from build123d import *
from OCP.BRepFilletAPI import BRepFilletAPI_MakeChamfer

# Parameters (mm, degrees)
BOSS_EXTRUDE1_DEPTH      = 25
BOSS_EXTRUDE1_DEPTH_BACK = 25
CUT_EXTRUDE1_DEPTH       = 25
BOSS_EXTRUDE3_DEPTH      = 20
CHAMFER2_SIZE            = 10
CHAMFER2_SIZE_2          = 0.5
SKETCH5_R                = 4
CUT_EXTRUDE4_DEPTH       = 20
SKETCH6_R                = 2.25
CUT_EXTRUDE5_DEPTH       = 20
CUT_EXTRUDE6_DEPTH       = 30
CUT_EXTRUDE6_DEPTH_BACK  = 20
SKETCH7_R                = 2.25
SKETCH8_R                = 4
CUT_EXTRUDE7_DEPTH       = 20
CUT_EXTRUDE10_DEPTH      = 10
CUT_EXTRUDE10_DEPTH_BACK = 10
SKETCH10_R               = 1.875
SKETCH10_9_R             = 3
SKETCH10_9_R_2           = 1.875
CUT_EXTRUDE11_DEPTH      = 20
CHAMFER3_START           = -141.531055451
CHAMFER3_DEPTH           = 67.531055451
CHAMFER4_SIZE            = 5
CHAMFER5_START           = 49.569652266
CHAMFER5_DEPTH           = 20.503333196
CHAMFER5_START_2         = -70.072985462
CHAMFER5_2_DEPTH         = 20.503333196


with BuildPart() as part:
    # Sketch1 → Boss-Extrude1 (new, two sides: drawn at the far end of the back side and taken through both)
    with BuildSketch(Plane(origin=(0, 0, 0), x_dir=(0, 0, -1), z_dir=(1, 0, 0)).offset(-BOSS_EXTRUDE1_DEPTH_BACK)):
        Polygon((-106.218311965, -85.648642757), (-56.372445278, -89.571597544), (-57.980856741, -110.008402885), (-53, -105), (-53, -65), (-73, -65), (-105.747557391, -79.667138755), align=None)
    extrude(amount=BOSS_EXTRUDE1_DEPTH + BOSS_EXTRUDE1_DEPTH_BACK)

    # Sketch2 → Cut-Extrude1 (cut)
    with BuildSketch(Plane(origin=(0, -65, 0), x_dir=(1, 0, 0), z_dir=(0, 1, 0))):
        Polygon((16.25, -106.218311965), (16.25, -73), (25, -63), (25, -106.218311965), align=None)
        Polygon((-25, -106.218311965), (-16.25, -106.218311965), (-16.25, -73), (-25, -63), align=None)
    extrude(amount=-CUT_EXTRUDE1_DEPTH, mode=Mode.SUBTRACT)

    # Sketch3 → Boss-Extrude3 (add)
    with BuildSketch(Plane(origin=(0, -93.429506703, 7.353061645), x_dir=(1, 0, 0), z_dir=(0, -0.9969173337331282, 0.07845909572784136))):
        Polygon((10.25, 99.170961297), (10.25, 49.170961297), (25, 49.170961297), (25, 55.819009733), (16.25, 65.849931718), (16.25, 99.170961297), align=None)
        Polygon((-10.25, 99.170961297), (-10.25, 49.170961297), (-25, 49.170961297), (-25, 55.819009733), (-16.25, 65.849931718), (-16.25, 99.170961297), align=None)
    extrude(amount=BOSS_EXTRUDE3_DEPTH)

    # Chamfer2
    chamfer2_edges_1 = [part.edges().sort_by_distance(p)[0] for p in [
        (17.625, -109.509944218, 57.941627193),
    ]]
    chamfer2_side_1 = [part.faces().sort_by_distance(p)[0] for p in [
        (17.625, -109.509159627, 57.951596366),
    ]]
    chamfer2_edges_2 = [part.edges().sort_by_distance(p)[0] for p in [
        (-17.625, -109.509944218, 57.941627193),
    ]]
    chamfer2_side_2 = [part.faces().sort_by_distance(p)[0] for p in [
        (-17.625, -109.509159627, 57.951596366),
    ]]
    chamfer2 = BRepFilletAPI_MakeChamfer(part.part.solid().wrapped)
    for e in chamfer2_edges_1:
        chamfer2.Add(CHAMFER2_SIZE - 0.0001, CHAMFER2_SIZE_2 - 0.0001, e.wrapped, chamfer2_side_1[0].wrapped)
    for e in chamfer2_edges_2:
        chamfer2.Add(CHAMFER2_SIZE - 0.0001, CHAMFER2_SIZE_2 - 0.0001, e.wrapped, chamfer2_side_2[0].wrapped)
    add(Compound.cast(chamfer2.Shape()), mode=Mode.REPLACE)  # a hair under: the kernel refuses the full size

    # Sketch5 → Cut-Extrude4 (cut)
    with BuildSketch(Plane(origin=(0, -87.448002701, 6.882307071), x_dir=(-1, 0, 0), z_dir=(0, -0.9969173337331282, 0.07845909572784136))):
        with Locations(Location((0, -61.670961297, 0), (0, 0, 90))):
            Circle(SKETCH5_R)
        with Locations(Location((0, -86.670961297, 0), (0, 0, 90))):
            Circle(SKETCH5_R)
    extrude(amount=-CUT_EXTRUDE4_DEPTH, mode=Mode.SUBTRACT)

    # Sketch6 → Cut-Extrude5 (cut)
    with BuildSketch(Plane(origin=(0, -87.448002701, 6.882307071), x_dir=(1, 0, 0), z_dir=(0, 0.9969173337331282, -0.07845909572784135))):
        with Locations(Location((0, -61.670961297, 0), (0, 0, 270))):
            Circle(SKETCH6_R)
        with Locations(Location((0, -86.670961297, 0), (0, 0, 270))):
            Circle(SKETCH6_R)
    extrude(amount=-CUT_EXTRUDE5_DEPTH, mode=Mode.SUBTRACT)

    # Sketch7 → Cut-Extrude6 (cut, two sides: drawn at the far end of the back side and taken through both)
    with BuildSketch(Plane(origin=(-10.25, 0, 0), x_dir=(0, 0, -1), z_dir=(1, 0, 0)).offset(-CUT_EXTRUDE6_DEPTH_BACK)):
        with Locations((-97.033729585, -96.402407052)):
            Circle(SKETCH7_R)
        with Locations((-77.09538291, -97.971588966)):
            Circle(SKETCH7_R)
    extrude(amount=CUT_EXTRUDE6_DEPTH + CUT_EXTRUDE6_DEPTH_BACK, mode=Mode.SUBTRACT)

    # Sketch8 → Cut-Extrude7 (cut)
    with BuildSketch(Plane.ZY.offset(16.25)):
        with Locations((77.09538291, -97.971588966)):
            Circle(SKETCH8_R)
    cut_extrude7 = extrude(amount=CUT_EXTRUDE7_DEPTH, mode=Mode.SUBTRACT)

    # Mirror1: Cut-Extrude7 across plane
    add(cut_extrude7.mirror(Plane.ZY), mode=Mode.SUBTRACT)

    # Sketch10 → Cut-Extrude10 (cut, two sides: drawn at the far end of the back side and taken through both)
    with BuildSketch(Plane(origin=(0, 0, 63), x_dir=(-1, 0, 0), z_dir=(0, 0, -1)).offset(-CUT_EXTRUDE10_DEPTH_BACK)):
        with Locations(Location((-20, -100, 0), (0, 0, 356.084777763))):
            Circle(SKETCH10_R)
        with Locations((-20, -80)):
            Circle(SKETCH10_R)
        with Locations(Location((20, -80, 0), (0, 0, 180))):
            Circle(SKETCH10_R)
        with Locations(Location((20, -100, 0), (0, 0, 183.915222237))):
            Circle(SKETCH10_R)
    extrude(amount=CUT_EXTRUDE10_DEPTH + CUT_EXTRUDE10_DEPTH_BACK, mode=Mode.SUBTRACT)

    # Sketch10<9> → Cut-Extrude11 (cut)
    # profile 1 of 4: a face of its own
    with BuildSketch(Plane(origin=(0, 0, 63), x_dir=(-1, 0, 0), z_dir=(0, 0, -1))):
        with Locations((20, -100)):
            Circle(SKETCH10_9_R)
        with Locations((20, -100)):
            Circle(SKETCH10_9_R_2, mode=Mode.SUBTRACT)
    # profile 2 of 4: a face of its own
    with BuildSketch(Plane(origin=(0, 0, 63), x_dir=(-1, 0, 0), z_dir=(0, 0, -1))):
        with Locations((20, -80)):
            Circle(SKETCH10_9_R)
        with Locations((20, -80)):
            Circle(SKETCH10_9_R_2, mode=Mode.SUBTRACT)
    # profile 3 of 4: a face of its own
    with BuildSketch(Plane(origin=(0, 0, 63), x_dir=(-1, 0, 0), z_dir=(0, 0, -1))):
        with Locations((-20, -80)):
            Circle(SKETCH10_9_R)
        with Locations((-20, -80)):
            Circle(SKETCH10_9_R_2, mode=Mode.SUBTRACT)
    # profile 4 of 4: a face of its own
    with BuildSketch(Plane(origin=(0, 0, 63), x_dir=(-1, 0, 0), z_dir=(0, 0, -1))):
        with Locations((-20, -100)):
            Circle(SKETCH10_9_R)
        with Locations((-20, -100)):
            Circle(SKETCH10_9_R_2, mode=Mode.SUBTRACT)
    extrude(amount=-CUT_EXTRUDE11_DEPTH, mode=Mode.SUBTRACT)

    # Chamfer3: read off the stored shape, not the designer's step
    # Chamfer3 outline → Chamfer3 (cut)
    with BuildSketch(Plane(origin=(0, 0, 0), x_dir=(1, 0, 0), z_dir=(0, 0.4087588305450842, -0.9126424373495983)).offset(CHAMFER3_START)):
        Polygon((-25, 43.232363798), (-25, 28), (-9.767636202, 28), align=None)
        Polygon((9.767636202, 28), (25, 28), (25, 43.232363798), align=None)
    extrude(amount=CHAMFER3_DEPTH, mode=Mode.SUBTRACT)

    # Chamfer4
    chamfer4_edges = [part.edges().sort_by_distance(p)[0] for p in [
        (-13.25, -105.586989432, 107.78749388),
        (13.25, -105.586989432, 107.78749388),
    ]]
    chamfer(chamfer4_edges, length=CHAMFER4_SIZE)

    # Chamfer5: read off the stored shape, not the designer's step
    # Chamfer5 outline → Chamfer5 (cut)
    with BuildSketch(Plane(origin=(0, 0, 0), x_dir=(0.7072170856964756, 0.7032116882513418, -0.0730569312637863), z_dir=(0.7069964594670781, -0.7034311334001396, 0.07307972950423045)).offset(CHAMFER5_START)):
        Polygon((-95.809344587, 42.345340215), (-95.562635623, 56.312202838), (-95.604662607, 58.691464219), (-95.627776424, 60), (-100, 60), (-100, 41), (-95.833108513, 41), align=None)
    extrude(amount=CHAMFER5_DEPTH, mode=Mode.SUBTRACT)

    # Chamfer5 2 outline → Chamfer5 2 (cut)
    with BuildSketch(Plane(origin=(0, 0, 0), x_dir=(0.7072170856964753, -0.7032116882513376, 0.0730569312638283), z_dir=(0.7069964594670783, 0.7034311334001349, -0.0730797295042724)).offset(CHAMFER5_START_2)):
        Polygon((95.809344587, -42.345340215), (95.562635623, -56.312202838), (95.604662607, -58.691464219), (95.627776424, -60), (100, -60), (100, -41), (95.833108513, -41), align=None)
    extrude(amount=CHAMFER5_2_DEPTH, mode=Mode.SUBTRACT)


solid = part.part
Input: part model. Units: mm. Frame: model coordinates. A direction names the side the tool comes from. Give positions to 0.01 mm unless a question says otherwise; leave off trailing zeros. Order: outer loops, then holes, each group sorted by start corner. A loop starts at its lowest first (then second) coordinate and runs counter-clockwise, first axis right, second up. Notation, with made-up numbers: M 87,-37 L 146,-37 A32 cw 146,-10 Z; hole C -1,27 d10. An arc over 180 degrees is marked long. Answer as a JSON object with one key per item and string values.
1. Pull-direction query (Z, two-part tool) for faces 1 (the cylindrical face through (-0.86, -83.43, 95.59)), 2 (the flat face through (-0.35, -107.539, 55.525)), 3 (the flat face through (20.686, -96.276, 68.529)); classes: +Z half, -Z half, draft (parallel to the pull), parting line (faces both ways), or undercut.
Result sheet:
{"face 1": "undercut", "face 2": "-Z half", "face 3": "+Z half"}
2. Cut plane A-A, the plane x = -6.5. Output: boundary loops of the cut face in (y, z), and give its area (3 significant figures).
Result sheet:
{"outline": "M -110.01,57.98 L -105,53 L -65,53 L -65,73 L -79.67,105.75 L -85.65,106.22 L -89.57,56.37 Z", "area": "1,030 mm²"}
3. Cut plane D-D, the plane z = 77. Output: boundary loops of the cut face in (x, y).
Result sheet:
{"outline": "M -16.25,-108.01 L -10.25,-108.01 L -10.25,-100.22 L -16.25,-100.22 Z; M -16.25,-95.72 L -10.25,-95.72 L -10.25,-87.95 L 10.25,-87.95 L 10.25,-95.72 L 16.25,-95.72 L 16.25,-72.27 L 11.25,-66.79 L -11.25,-66.79 L -16.25,-72.27 Z; M 10.25,-108.01 L 16.25,-108.01 L 16.25,-100.22 L 10.25,-100.22 Z"}
4. Cut plane B-B, the plane z = 61. Output: boundary loops of the cut face in (x, y) (3 decimals).
Result sheet:
{"outline": "M -25,-104.577 L -20,-109.618 L -10.25,-109.618 L -10.25,-89.207 L 10.25,-89.207 L 10.25,-109.618 L 20,-109.618 L 25,-104.577 L 25,-74.692 L 16.155,-65 L -16.155,-65 L -25,-74.692 Z; hole C -20,-100 d3.75; hole C -20,-80 d3.75; hole C 20,-100 d3.75; hole C 20,-80 d3.75"}
5. Reachability of faces 4 (the flat face through (20.564, -83.761, 68.07)), 5 (the cylindrical face through (17.14, -79.1, 66.49)), 6 (the flat face through (-20.564, -83.761, 68.07)), 7 (the flat face through (-13.973, -107.333, 85.601)) from +Z, -Z, +X, -X, +Y, -Y: full face, straight path, thin tool, end or side. Return the list, or none.
Result sheet:
{"face 4": "+Z, +X, +Y", "face 5": "+Z", "face 6": "+Z, -X, +Y", "face 7": "+Z, +X, -X, -Y"}
6. First-contact query: P1, Ø3, axis at x = 20, y = -100, coming from the -Z side; P2, Ø8, axis at y = -92, z = 80.5, coming from the -X side; P3, Ø8, axis at x = 2, z = 94, coming from the +Y side; P4, Ø7, axis at x = 20, y = -80, coming from the +Z side. Flat tips, straight axial feed; report the tip coordinate or a pass-through.
Result sheet:
{"P1": "through", "P2": "x = -16.25", "P3": "y = -72.69", "P4": "z = 72.71"}
7. Ray query, line 1 (X direction, y = -100, z = 55.5) (3 decimals); line 2 (X direction, y = -100, z = 57.25) (3 decimals); line 3 (Y direction, x = -20, z = 65). Return the intervals inside material, ascending. Write a range as [from, to].
Result sheet:
{"line 1": "[-25, -21.875], [-18.125, 18.125], [21.875, 25]", "line 2": "[-25, -21.875], [-18.125, -10.25], [10.25, 18.125], [21.875, 25]", "line 3": "[-109.1, -103], [-97, -83], [-77, -71]"}
8. Cut plane C-C, the plane x = -14.5. State how many separate pieces and enclosed holes the cut face has, and give its area (3 significant figures).
Result sheet:
{"separate pieces": "1", "enclosed holes": "2", "area": "1,860 mm²"}
